Input: part model. Units: mm. Frame: model coordinates. A direction names the side the tool comes from. Coordinates: 2 decimals unless noted, no trailing zeros. Loops run counter-clockwise (first coordinate to the right, second up) from the corner with the lowest first, then second, coordinate; pieces in that order, holes last. Notation, with made-up numbers: (84, 56) -> (140, 56) arc R30 ccw to (140, 79) -> close; hole circle Ø1 at (-5.75, -22.75). An arc over 180 degrees is marked (long way). Answer as a JSON object with one key per item and string values.
from build123d import *

# Parameters (mm, degrees)
F1_DEPTH     = 110
F3_DEPTH     = 9.14
F5_DEPTH     = 9.14
F7_DEPTH     = 9.14
F8_T1_DEPTH  = 8.75
F8_T3_DEPTH  = 8.75
F8_T5_DEPTH  = 8.75
F8_T7_DEPTH  = 8.75
F8_T9_DEPTH  = 8.75
F8_T11_DEPTH = 8.6204005009
F9_R         = 0.5


# Not quite as in the source:
# - a fillet or chamfer that OpenCascade refuses, or shapes differently, is made with other operations: its cross-section is extruded or revolved along the edge and cut away or added


with BuildPart() as f1:
    # F0 (on Top) → F1 (new body)
    with BuildSketch(Plane.XY):
        Polygon((2.5, 1.443375673), (0, 2.8867513459), (-2.5, 1.443375673), (-2.5, -1.443375673), (0, -2.8867513459), (2.5, -1.443375673), align=None)
        Polygon((-1.5, 0.8660254038), (0, 1.7320508076), (1.5, 0.8660254038), (1.5, -0.8660254038), (0, -1.7320508076), (-1.5, -0.8660254038), align=None, mode=Mode.SUBTRACT)
    extrude(amount=F1_DEPTH)

    # F2 (on face) → F3 (join)
    with BuildSketch(Plane(origin=(-1.25, -2.1650635095, 0), x_dir=(0.8660254038, -0.5, 0), z_dir=(-0.5, -0.8660254038, 0))):
        Polygon((-1.443375673, 43.018942656), (1.443375673, 53.018942656), (1.443375673, 55.018942656), (-1.443375673, 45.018942656), align=None)
        Polygon((1.443375673, 31.018942656), (1.443375673, 33.018942656), (-1.443375673, 23.4446715784), (-1.443375673, 21.4446715784), align=None)
        Polygon((1.443375673, 9.4446715784), (1.443375673, 11.4446715784), (-1.443375673, 1.8704005009), (-1.443375673, 0), (-1.4042999537, 0), align=None)
    extrude(amount=F3_DEPTH)

    # F4 (on face) → F5 (join)
    with BuildSketch(Plane(origin=(-1.25, 2.1650635095, 0), x_dir=(-0.8660254038, -0.5, 0), z_dir=(-0.5, 0.8660254038, 0))):
        Polygon((-1.443375673, 43.018942656), (1.443375673, 53.018942656), (1.443375673, 55.018942656), (-1.443375673, 45.018942656), align=None)
        Polygon((1.443375673, 31.018942656), (1.443375673, 33.018942656), (-1.443375673, 23.4446715784), (-1.443375673, 21.4446715784), align=None)
        Polygon((1.443375673, 9.4446715784), (1.443375673, 11.4446715784), (-1.443375673, 1.8704005009), (-1.443375673, 0), (-1.4042999537, 0), align=None)
    extrude(amount=F5_DEPTH)

    # F6 (on face) → F7 (join)
    with BuildSketch(Plane.YZ.offset(2.5)):
        Polygon((-1.443375673, 43.018942656), (1.443375673, 53.018942656), (1.443375673, 55.018942656), (-1.443375673, 45.018942656), align=None)
        Polygon((1.443375673, 31.018942656), (1.443375673, 33.018942656), (-1.443375673, 23.4446715784), (-1.443375673, 21.4446715784), align=None)
        Polygon((1.443375673, 9.4446715784), (1.443375673, 11.4446715784), (-1.443375673, 1.8704005009), (-1.443375673, 0), (-1.4042999537, 0), align=None)
    extrude(amount=F7_DEPTH)

    # F8: fillet of radius 1 on 18 edges, made by hand

    # F8_s2 → F8_t1 (cut)
    with BuildSketch(Plane.XY.offset(40.518942656)):
        with BuildLine():
            ThreePointArc((-6.57, -8.4928224598), (-6.6699004225, -9.2516415049), (-6.2039745962, -9.8588478636))
            Line((-6.2039745962, -9.8588478636), (-7.07, -9.3588478636))
            Line((-7.07, -9.3588478636), (-6.57, -8.4928224598))
        make_face()
        with BuildLine():
            ThreePointArc((11.64, -0.443375673), (11.3471067812, -1.1504824542), (10.64, -1.443375673))
            Line((10.64, -1.443375673), (11.64, -1.443375673))
            Line((11.64, -1.443375673), (11.64, -0.443375673))
        make_face()
        with BuildLine():
            ThreePointArc((-4.07, 9.9361981328), (-4.6772063587, 10.402123959), (-5.4360254038, 10.3022235365))
            Line((-5.4360254038, 10.3022235365), (-4.57, 10.8022235365))
            Line((-4.57, 10.8022235365), (-4.07, 9.9361981328))
        make_face()
    extrude(amount=F8_T1_DEPTH, mode=Mode.SUBTRACT)

    # F8_s4 → F8_t3 (cut)
    with BuildSketch(Plane.XY.offset(48.768942656)):
        with BuildLine():
            ThreePointArc((-4.07, -9.9361981328), (-4.6772063587, -10.402123959), (-5.4360254038, -10.3022235365))
            Line((-5.4360254038, -10.3022235365), (-4.57, -10.8022235365))
            Line((-4.57, -10.8022235365), (-4.07, -9.9361981328))
        make_face()
        with BuildLine():
            ThreePointArc((10.64, 1.443375673), (11.3471067812, 1.1504824542), (11.64, 0.443375673))
            Line((11.64, 0.443375673), (11.64, 1.443375673))
            Line((11.64, 1.443375673), (10.64, 1.443375673))
        make_face()
        with BuildLine():
            ThreePointArc((-6.2039745962, 9.8588478636), (-6.6699004225, 9.2516415049), (-6.57, 8.4928224598))
            Line((-6.57, 8.4928224598), (-7.07, 9.3588478636))
            Line((-7.07, 9.3588478636), (-6.2039745962, 9.8588478636))
        make_face()
    extrude(amount=F8_T3_DEPTH, mode=Mode.SUBTRACT)

    # F8_s6 → F8_t5 (cut)
    with BuildSketch(Plane.XY.offset(26.768942656)):
        with BuildLine():
            ThreePointArc((-4.07, -9.9361981328), (-4.6772063587, -10.402123959), (-5.4360254038, -10.3022235365))
            Line((-5.4360254038, -10.3022235365), (-4.57, -10.8022235365))
            Line((-4.57, -10.8022235365), (-4.07, -9.9361981328))
        make_face()
        with BuildLine():
            ThreePointArc((10.64, 1.443375673), (11.3471067812, 1.1504824542), (11.64, 0.443375673))
            Line((11.64, 0.443375673), (11.64, 1.443375673))
            Line((11.64, 1.443375673), (10.64, 1.443375673))
        make_face()
        with BuildLine():
            ThreePointArc((-6.2039745962, 9.8588478636), (-6.6699004225, 9.2516415049), (-6.57, 8.4928224598))
            Line((-6.57, 8.4928224598), (-7.07, 9.3588478636))
            Line((-7.07, 9.3588478636), (-6.2039745962, 9.8588478636))
        make_face()
    extrude(amount=F8_T5_DEPTH, mode=Mode.SUBTRACT)

    # F8_s8 → F8_t7 (cut)
    with BuildSketch(Plane.XY.offset(18.9446715784)):
        with BuildLine():
            ThreePointArc((-6.57, -8.4928224598), (-6.6699004225, -9.2516415049), (-6.2039745962, -9.8588478636))
            Line((-6.2039745962, -9.8588478636), (-7.07, -9.3588478636))
            Line((-7.07, -9.3588478636), (-6.57, -8.4928224598))
        make_face()
        with BuildLine():
            ThreePointArc((11.64, -0.443375673), (11.3471067812, -1.1504824542), (10.64, -1.443375673))
            Line((10.64, -1.443375673), (11.64, -1.443375673))
            Line((11.64, -1.443375673), (11.64, -0.443375673))
        make_face()
        with BuildLine():
            ThreePointArc((-4.07, 9.9361981328), (-4.6772063587, 10.402123959), (-5.4360254038, 10.3022235365))
            Line((-5.4360254038, 10.3022235365), (-4.57, 10.8022235365))
            Line((-4.57, 10.8022235365), (-4.07, 9.9361981328))
        make_face()
    extrude(amount=F8_T7_DEPTH, mode=Mode.SUBTRACT)

    # F8_s10 → F8_t9 (cut)
    with BuildSketch(Plane.XY.offset(5.1946715784)):
        with BuildLine():
            ThreePointArc((-5.4360254038, -10.3022235365), (-4.6772063587, -10.402123959), (-4.07, -9.9361981328))
            Line((-4.07, -9.9361981328), (-4.57, -10.8022235365))
            Line((-4.57, -10.8022235365), (-5.4360254038, -10.3022235365))
        make_face()
        with BuildLine():
            ThreePointArc((10.64, 1.443375673), (11.3471067812, 1.1504824542), (11.64, 0.443375673))
            Line((11.64, 0.443375673), (11.64, 1.443375673))
            Line((11.64, 1.443375673), (10.64, 1.443375673))
        make_face()
        with BuildLine():
            ThreePointArc((-6.2039745962, 9.8588478636), (-6.6699004225, 9.2516415049), (-6.57, 8.4928224598))
            Line((-6.57, 8.4928224598), (-7.07, 9.3588478636))
            Line((-7.07, 9.3588478636), (-6.2039745962, 9.8588478636))
        make_face()
    extrude(amount=F8_T9_DEPTH, mode=Mode.SUBTRACT)

    # F8_s12 → F8_t11 (cut)
    with BuildSketch(Plane.XY.offset(-2.5)):
        with BuildLine():
            ThreePointArc((-6.57, -8.4928224598), (-6.6699004225, -9.2516415049), (-6.2039745962, -9.8588478636))
            Line((-6.2039745962, -9.8588478636), (-7.07, -9.3588478636))
            Line((-7.07, -9.3588478636), (-6.57, -8.4928224598))
        make_face()
        with BuildLine():
            ThreePointArc((11.64, -0.443375673), (11.3471067812, -1.1504824542), (10.64, -1.443375673))
            Line((10.64, -1.443375673), (11.64, -1.443375673))
            Line((11.64, -1.443375673), (11.64, -0.443375673))
        make_face()
        with BuildLine():
            ThreePointArc((-4.07, 9.9361981328), (-4.6772063587, 10.402123959), (-5.4360254038, 10.3022235365))
            Line((-5.4360254038, 10.3022235365), (-4.57, 10.8022235365))
            Line((-4.57, 10.8022235365), (-4.07, 9.9361981328))
        make_face()
    extrude(amount=F8_T11_DEPTH, mode=Mode.SUBTRACT)

    # F9
    f9_edges = [f1.edges().sort_by_distance(p)[0] for p in [
        (1.25, -2.165064, 0),
        (-1.23308, -2.174832, 0),
        (-2.5, 0, 0),
        (-1.26692, 2.155295, 0),
        (1.25, 2.165064, 0),
        (2.5, 0.019538, 0),
    ]]
    fillet(f9_edges, radius=F9_R)


solid = f1.part
1. Section query B-B (y = -6). Return loops of the section in (x, z).
Reply:
{"outline": "(-5.13, 0) -> (-5.09, 0) -> (-1.8, 9.44) -> (-1.8, 11.44) -> (-5.13, 1.87) -> close; (-5.13, 21.44) -> (-1.8, 31.02) -> (-1.8, 33.02) -> (-5.13, 23.44) -> close; (-5.13, 43.02) -> (-1.8, 53.02) -> (-1.8, 55.02) -> (-5.13, 45.02) -> close"}
2. Section query A-A (z = 70.5). Return loops of the section in (x, y), plus the area to 3 significant figures.
Reply:
{"outline": "(-2.5, -1.44) -> (0, -2.89) -> (2.5, -1.44) -> (2.5, 1.44) -> (0, 2.89) -> (-2.5, 1.44) -> close; hole (-1.5, -0.87) -> (0, -1.73) -> (1.5, -0.87) -> (1.5, 0.87) -> (0, 1.73) -> (-1.5, 0.87) -> close", "area": "13.9 mm2"}
3. Section query C-C (z = 54). Return loops of the section in (x, y).
Reply:
{"outline": "(-6.67, 9.25) arc R1 ccw to (-6.57, 8.49) -> (-2.5, 1.44) -> (-2.5, -1.44) -> (-0.25, -2.74) -> (-4.68, -10.4) arc R1 ccw to (-4.07, -9.94) -> (0, -2.89) -> (2.5, -1.44) -> (2.5, 1.15) -> (11.35, 1.15) arc R1 ccw to (10.64, 1.44) -> (2.5, 1.44) -> (0, 2.89) -> (-2.25, 1.59) -> close; hole (-1.5, -0.87) -> (0, -1.73) -> (1.5, -0.87) -> (1.5, 0.87) -> (0, 1.73) -> (-1.5, 0.87) -> close"}
4. Access query for faces 1 (the face through (-0.67, -2.5, 2.92)), 2 (the face through (-1.267, -2.155, 16.241)), 3 (the face through (-2.5, 0, 54)). Directions: +Z, -Z, +X, -X, +Y, -Y. A direction counts if a zero-diameter tool reaches every point of the face in a straight line with its end or side. Return the directions, or none.
Reply:
{"face 1": "-Z, -Y", "face 2": "none", "face 3": "+Z, -Z, -X"}
5. Mould query, pull axis Y, two halves, no side actions, for faces 4 (the face through (-4.507, -4.919, 44.033)), 5 (the face through (-1.75, 5.92, 0.95)), 6 (the face through (7.01, 0.02, 6.72)). Classes: pulls with the +Y half, pulls with the -Y half, needs draft (parallel to the pull), parting line crosses it, or undercut.
Reply:
{"face 4": "undercut", "face 5": "pulls with the +Y half", "face 6": "pulls with the -Y half"}
6. Line query: line 1 along X through (y, z) = (-0.5, 38.5); line 2 along Y through (x, z) = (1, 20); line 3 along X through (y, z) = (-1.5, 13). Output: solid intervals per line, ascending.
Reply:
{"line 1": "x = -2.5 to -1.5, 1.5 to 2.5", "line 2": "y = -2.31 to -1.15, 1.15 to 2.31", "line 3": "x = -2.4 to -0.4, 0.4 to 2.4"}
7. Pin query (flat end, axial travel): P1, Ø2, axis at x = 0.5, z = 63.5, coming from the -Y side; P2, Ø0.6, axis at x = 5, z = 10, coming from the +Y side; P3, Ø1.4, axis at y = 0.5, z = 53, coming from the +X side. Return the tip coordinate at first contact, or that it passes through.
Reply:
{"P1": "stops at y = -2.89", "P2": "stops at y = 1.44", "P3": "stops at x = 11.62"}
